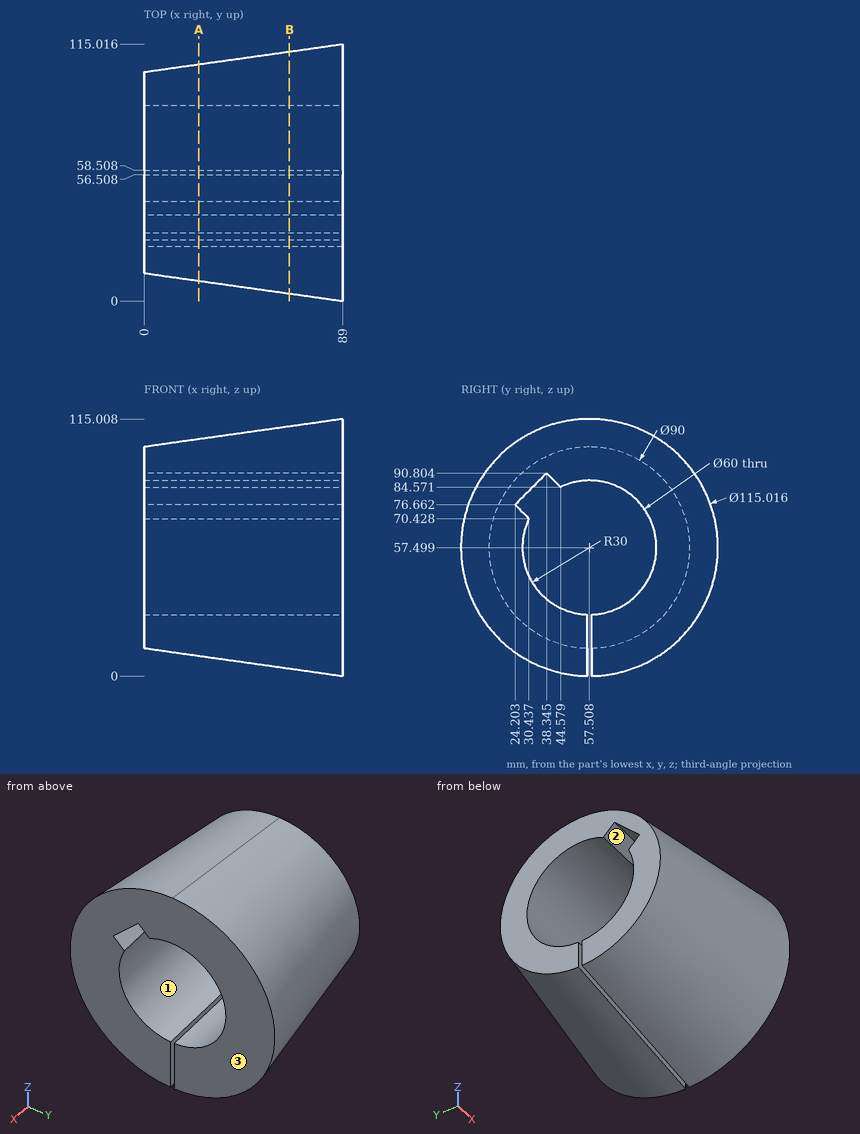
Check sheet for the drawn part. Datum: minimum x, y, z corner. Units: mm. Round coordinates to 2 decimals unless told otherwise and drop trailing zeros. Write each loop counter-clockwise with the first axis right and the second up, starting at its lowest first coordinate (ties: lowest second). Pieces come first, ordered by that corner, then holes. Notation, with made-up numbers: (14.25, 71.25) - (61.25, 71.25) arc R19 ccw to (61.25, 91.25) - close; hole circle Ø7 at (47.25, 33.25). An arc over 180 degrees is marked (long way). Write each question's results on one line, items separated by ' | '.
(1) Sectioned sample at B-B, the plane x = 65. Enter the section's corners in (y, z) (1 decimal), plus the area to 3 significant figures.
Computed:
outline: (24.2, 76.7) - (38.3, 90.8) - (44.6, 84.6) arc R30 cw (long way) to (58.5, 27.5) - (58.5, 3.4) arc R54.1 ccw (long way) to (56.5, 3.4) - (56.5, 27.5) arc R30 cw to (30.4, 70.4) - close | area: 6,180 mm^2
(2) Depth check by flat-ended pin: pin 1 Ø12 at (x, y) = (14.5, 69) entering from -Z; pin 2 Ø12 at (x, z) = (29, 102.5) entering from -Y (1 decimal); pin 3 Ø5 at (x, z) = (37, 86.5) entering from +Y. Enter the tip coordinate at first touch or a pass-through.
Computed:
pin 1: stops at z = 10.42 | pin 2: stops at y = 27.6 | pin 3: stops at y = 100.2
(3) Sectioned sample at A-A, the plane x = 24.5. Enter the section's corners in (y, z) (1 decimal).
Computed:
outline: (24.2, 76.7) - (38.3, 90.8) - (44.6, 84.6) arc R30 cw (long way) to (58.5, 27.5) - (58.5, 9.1) arc R48.4 ccw (long way) to (56.5, 9.1) - (56.5, 27.5) arc R30 cw to (30.4, 70.4) - close
(4) Draft check along Y on the marked faces 1, 2 and 3. Enter one of: pulls with the +Y half, pulls with the -Y half, needs draft (parallel to the pull), parting line crosses it, or undercut.
Computed:
face 1: undercut | face 2: undercut | face 3: needs draft
(5) Thickness scan on probe 1 along Y at (x, z) = (24.5, 23) (1 decimal); probe 2 along Z at (x, y) = (11.5, 25) (1 decimal); probe 3 along Z at (x, y) = (77, 37.5) (1 decimal). Record the ranges inside material, lowest first. Write a range as from..to.
Computed:
probe 1: y = 23.5..56.5, 58.5..91.5 | probe 2: z = 24.1..75.9, 77.5..90.9 | probe 3: z = 5.4..35.1, 90..109.6
